The model under review builds one solid part; all positions refer to its coordinate system, in mm. Coordinates: 2 decimals unless noted, no trailing zeros. Write each loop counter-clockwise with the first axis right and the second up, starting at its lowest first coordinate (ties: lowest second). Pieces come first, ordered by that corner, then holes. Notation, with made-up numbers: M 5,32.5 L 31,32.5 A28 ccw 31,58.5 Z; hole C -1,-29.5 d10. An arc over 180 degrees is marked long. Answer as a JSON object with one key per item and string values.
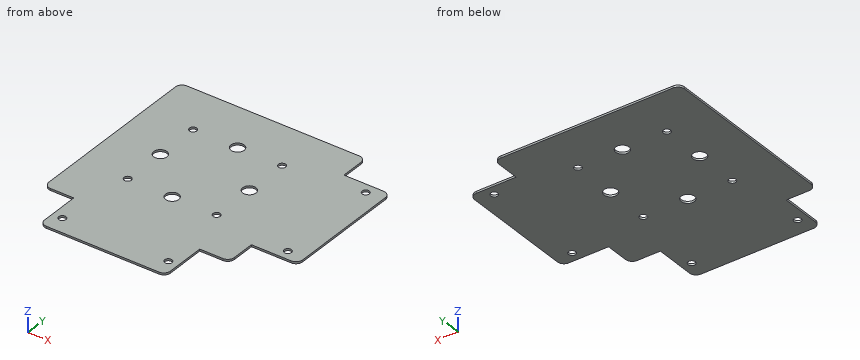
```python
from build123d import *

# Parameters (mm, degrees)
F0_W     = 35
F0_H     = 95
F0_R     = 2.75
F0_W_2   = 95
F0_H_2   = 35
F1_DEPTH = 1.5
F2_R     = 2.75
F2_R_2   = 5
F3_DEPTH = 1.501
F4_R     = 5
F5_R     = 5


with BuildPart() as f1:
    # F0 (on Top) → F1 (new body)
    with BuildSketch(Plane.XY):
        Polygon((70, 70), (-70, 70), (-70, -70), (-47.5, -70), (47.5, -70), (70, -70), (70, -47.5), (70, 47.5), align=None)
        with Locations((87.5, 0)):
            Rectangle(F0_W, F0_H)
        with Locations((92, -40)):
            Circle(F0_R, mode=Mode.SUBTRACT)
        with Locations((92, 40)):
            Circle(F0_R, mode=Mode.SUBTRACT)
        with Locations((0, -87.5)):
            Rectangle(F0_W_2, F0_H_2)
        with Locations((-40, -92)):
            Circle(F0_R, mode=Mode.SUBTRACT)
        with Locations((40, -92)):
            Circle(F0_R, mode=Mode.SUBTRACT)
    extrude(amount=F1_DEPTH)

    # F2 (on face) → F3 (cut, through all)
    with BuildSketch(Plane.XY.offset(1.5)):
        with Locations((-33.587572, -33.587572)):
            Circle(F2_R)
        with Locations((33.587572, -33.587572)):
            Circle(F2_R)
        with Locations((-33.587572, 33.587572)):
            Circle(F2_R)
        with Locations((33.587572, 33.587572)):
            Circle(F2_R)
        with Locations((0, -33.587572)):
            Circle(F2_R_2)
        with Locations((33.587572, 0)):
            Circle(F2_R_2)
        with Locations((-33.587572, 0)):
            Circle(F2_R_2)
        with Locations((0, 33.587572)):
            Circle(F2_R_2)
    extrude(amount=-F3_DEPTH, mode=Mode.SUBTRACT)

    # F4
    f4_edges = [f1.edges().sort_by_distance(p)[0] for p in [
        (70, -70, 0.75),
        (-70, -70, 0.75),
        (70, 70, 0.75),
        (-70, 70, 0.75),
    ]]
    fillet(f4_edges, radius=F4_R)

    # F5
    f5_edges = [f1.edges().sort_by_distance(p)[0] for p in [
        (-47.5, -105, 0.75),
        (47.5, -105, 0.75),
        (105, -47.5, 0.75),
        (105, 47.5, 0.75),
    ]]
    fillet(f5_edges, radius=F5_R)


solid = f1.part
```
(1) Wall thickness on line 1 along Y through (x, z) = (92, 0.85); line 2 along X through (y, z) = (-2.5, 1); line 3 along X through (y, z) = (3.5, 0.85): over which ranges is each line inside the solid? List them lowest first. Write a range as from..to.
Results list:
{"line 1": "-47.5..-42.75, -37.25..37.25, 42.75..47.5", "line 2": "-70..-37.92, -29.26..29.26, 37.92..105", "line 3": "-70..-37.16, -30.02..30.02, 37.16..105"}
(2) Add section A-A on y = 0. Give the boundary of the cut face in (x, z).
Results list:
{"outline": "M -70,0 L -38.59,0 L -38.59,1.5 L -70,1.5 Z; M -28.59,0 L 28.59,0 L 28.59,1.5 L -28.59,1.5 Z; M 38.59,0 L 105,0 L 105,1.5 L 38.59,1.5 Z"}
(3) Add section C-C on z = 0.75. Count the separate pieces of the cut face and the enclosed holes in it, and give its area (3 significant figures).
Results list:
{"separate pieces": "1", "enclosed holes": "12", "area": "25,700 mm²"}
(4) Add section B-B on x = 92. Give the boundary of the cut face in (y, z).
Results list:
{"outline": "M -47.5,0 L -42.75,0 L -42.75,1.5 L -47.5,1.5 Z; M -37.25,0 L 37.25,0 L 37.25,1.5 L -37.25,1.5 Z; M 42.75,0 L 47.5,0 L 47.5,1.5 L 42.75,1.5 Z"}
(5) For pin 1 Ø9 at (x, y) = (33.59, 0) entering from +Z; pin 2 Ø0.8 at (x, z) = (-57.5, 1) entering from -Y; pin 3 Ø0.8 at (x, z) = (81.5, 0.5) entering from -Y; pin 4 Ø0.8 at (y, z) = (60, 1) entering from +X, all flat-tipped, find the tip position at first contact; note any pin that passes through.
Results list:
{"pin 1": "through", "pin 2": "y = -70", "pin 3": "y = -47.5", "pin 4": "x = 70"}
(6) Add section D-D on x = 59. Give the boundary of the cut face in (y, z).
Results list:
{"outline": "M -70,0 L 70,0 L 70,1.5 L -70,1.5 Z"}
